Verification items for the finished model (mm, model axes). A direction names the side the tool comes from. Give positions to 0.01 mm unless a question says otherwise; leave off trailing zeros. Write each loop counter-clockwise with the first axis right and the second up, starting at its lowest first coordinate (ties: lowest second). Pieces come first, ordered by that corner, then holes. Notation, with made-up numbers: (-19, -1) -> (22, -1) arc R18 cw to (22, 12) -> close; hole circle Ø3 at (3.25, 85.5). An arc over 180 degrees is marked (long way). Answer as CSV lines item,"result".
```python
from build123d import *

# Parameters (mm, degrees)
F0_R     = 28.232887
F1_DEPTH = 114.3
F2_T     = -2.54
F3_W     = 40.50754
F3_H     = 80.898837
F4_DEPTH = 12.7


with BuildPart() as f1:
    # F0 (on Front) → F1 (new body)
    with BuildSketch(Plane.XZ):
        with Locations((35.670944, 42.30497)):
            Circle(F0_R)
    extrude(amount=F1_DEPTH)

    # F2
    f2_openings = [f1.faces().sort_by_distance(p)[0] for p in [
        (35.670944, -114.3, 42.30497),
    ]]
    offset(amount=F2_T, openings=f2_openings)

    # F3 (on Right) → F4 (join)
    with BuildSketch(Plane.YZ):
        with Locations((-82.380377, 24.268664)):
            Rectangle(F3_W, F3_H)
    extrude(amount=F4_DEPTH)


solid = f1.part
```
1) Section check B-B (x = 46.5). Record the boundary of the cut face in (y, z).
Reported:
outline,"(-114.3, 16.23) -> (0, 16.23) -> (0, 68.38) -> (-114.3, 68.38) -> (-114.3, 65.6) -> (-2.54, 65.6) -> (-2.54, 19.01) -> (-114.3, 19.01) -> close"
2) Section check A-A (y = -93). Record the boundary of the cut face in (x, z).
Reported:
outline,"(0, -16.18) -> (12.7, -16.18) -> (12.7, 25.89) arc R28.23 ccw (long way) to (12.7, 58.72) -> (12.7, 64.72) -> (0, 64.72) -> close; hole (12.7, 30.8) arc R25.69 ccw (long way) to (12.7, 53.81) -> close"
3) Section check D-D (z = 37). Record the boundary of the cut face in (x, y).
Reported:
outline,"(0, -102.63) -> (7.94, -102.63) -> (7.94, -114.3) -> (10.53, -114.3) -> (10.53, -102.63) -> (12.7, -102.63) -> (12.7, -62.13) -> (10.53, -62.13) -> (10.53, -2.54) -> (60.81, -2.54) -> (60.81, -114.3) -> (63.4, -114.3) -> (63.4, 0) -> (7.94, 0) -> (7.94, -62.13) -> (0, -62.13) -> close"
4) Section check C-C (z = 10.5). Record the boundary of the cut face in (x, y).
Reported:
outline,"(0, -102.63) -> (12.7, -102.63) -> (12.7, -62.13) -> (0, -62.13) -> close"
5) Draft check along Z on faces 4 (the flat face through (6, -83, 64.718)), 5 (the flat face through (35, 0, 43)), 6 (the flat face through (12, -102.634, 42)). Enter one of: +Z half, -Z half, draft (parallel to the pull), parting line (faces both ways), or undercut.
Reported:
face 4,"+Z half"
face 5,"draft"
face 6,"undercut"
6) Scan lines: line 1 along X through (y, z) = (-102, 42.5); line 2 along X through (y, z) = (-74, 12.5); line 3 along Y through (x, z) = (8.5, 1). Record each from-to range of solid material in increasing order.
Reported:
line 1,"0 to 12.7, 61.36 to 63.9"
line 2,"0 to 12.7"
line 3,"-102.63 to -62.13"
7) Tool access check on faces 1 (the flat face through (12.7, -83, 5)), 2 (the flat face through (12.7, -83, 42)), 3 (the flat face through (12, -62.127, 42)). Record the directions out of +Z, -Z, +X, -X, +Y, -Y that give a thin tool (end or side, any length) a straight path to the whole face; none if there is none.
Reported:
face 1,"-Z, +Y, -Y"
face 2,"-Y"
face 3,"none"
8) Depth check by flat-ended pin: pin 1 (6.5 mm diameter, centred on x = 3.5, z = 19.5, fed in from +Y); pin 2 (6.5 mm diameter, centred on x = 5.5, y = -78.5, fed in from +Z); pin 3 (0.8 mm diameter, centred on x = 11.5, z = 40.5, fed in from -Y). Enter the tip coordinate at first touch or a pass-through.
Reported:
pin 1,"y = -62.13"
pin 2,"z = 64.72"
pin 3,"y = -102.63"
